```python
from build123d import *

# Parameters (mm, degrees)
SKETCH1_R           = 4.15
BOSS_EXTRUDE1_DEPTH = 27
BOSS_EXTRUDE2_DEPTH = 49
SKETCH3_W           = 7.137224295
SKETCH3_H           = 7.139279227
BOSS_EXTRUDE3_DEPTH = 49
SKETCH4_R           = 2
CUT_EXTRUDE1_DEPTH  = 51
FILLET1_R           = 3
SKETCH5_W           = 7.156865167
SKETCH5_H           = 37
CUT_EXTRUDE2_DEPTH  = 7.139279
SKETCH7_W           = 36.574972609
SKETCH7_H           = 48.532858444
CUT_EXTRUDE3_DEPTH  = 51
SKETCH8_W           = 4
SKETCH8_H           = 11
BOSS_EXTRUDE4_DEPTH = 49
SKETCH10_R          = 3.175
CUT_EXTRUDE4_DEPTH  = 49


with BuildPart() as part:
    # Sketch1 → Boss-Extrude1 (new body)
    with BuildSketch(Plane(origin=(0, 0, 0), x_dir=(1, 0, 0), z_dir=(0, 1, 0))):
        with BuildLine():
            Line((-6.5, 48.7), (-6.5, 0))
            ThreePointArc((-6.5, 0), (0, -6.5), (6.5, 0))
            Line((6.5, 0), (6.5, 48.7))
            ThreePointArc((6.5, 48.7), (0, 55.2), (-6.5, 48.7))
        make_face()
        with Locations(Location((0, 0, 0), (0, 0, 270))):  # turned: the seam where the file's is
            Circle(SKETCH1_R, mode=Mode.SUBTRACT)
        with Locations(Location((0, 48.7, 0), (0, 0, 270))):  # turned: the seam where the file's is
            Circle(SKETCH1_R, mode=Mode.SUBTRACT)
    extrude(amount=BOSS_EXTRUDE1_DEPTH)

    # Sketch2 → Boss-Extrude2 (add)
    with BuildSketch(Plane.XY):
        with BuildLine():
            Line((6.5, 27), (6.5, 0))
            Line((6.5, 0), (15.568570347, -6.685733343))
            ThreePointArc((15.568570347, -6.685733343), (43.70403904, -11.497551626), (60.435084664, 11.628846841))
            Line((60.435084664, 11.628846841), (62.638339389, 10.782838022))
            Line((62.638339389, 10.782838022), (62.638339389, 13.5))
            Line((62.638339389, 13.5), (57.5, 13.5))
            ThreePointArc((57.5, 13.5), (26.437253933, -9.437253933), (13.656865167, 27))
            Line((13.656865167, 27), (6.5, 27))
        make_face()
    extrude(amount=-BOSS_EXTRUDE2_DEPTH)

    # Sketch3 → Boss-Extrude3 (add)
    with BuildSketch(Plane.XY):
        with Locations((10.068612148, 30.569639614)):
            Rectangle(SKETCH3_W, SKETCH3_H)
    extrude(amount=-BOSS_EXTRUDE3_DEPTH)

    # Sketch4 → Cut-Extrude1 (cut)
    with BuildSketch(Plane.XY):
        with Locations((10.068612147, 30.569639613)):
            Circle(SKETCH4_R)
    extrude(amount=-CUT_EXTRUDE1_DEPTH, mode=Mode.SUBTRACT)

    # Fillet1
    fillet1_edges = [part.edges().sort_by_distance(p)[0] for p in [
        (6.5, 34.139279227, -24.5),
        (13.637224295, 34.139279227, -24.5),
    ]]
    fillet(fillet1_edges, radius=FILLET1_R)

    # Sketch5 → Cut-Extrude2 (cut)
    with BuildSketch(Plane(origin=(0, 34.139279227, 0), x_dir=(1, 0, 0), z_dir=(0, 1, 0))):
        with Locations((10.078432583, 24.5)):
            Rectangle(SKETCH5_W, SKETCH5_H)
    extrude(amount=-CUT_EXTRUDE2_DEPTH, mode=Mode.SUBTRACT)

    # Sketch7 → Cut-Extrude3 (cut)
    with BuildSketch(Plane.XY):
        with Locations((51.787486304, 3.889520552)):
            Rectangle(SKETCH7_W, SKETCH7_H)
    extrude(amount=-CUT_EXTRUDE3_DEPTH, mode=Mode.SUBTRACT)

    # Sketch8 → Boss-Extrude4 (add)
    with BuildSketch(Plane.XY):
        with Locations((31.5, -16)):
            Rectangle(SKETCH8_W, SKETCH8_H)
    extrude(amount=-BOSS_EXTRUDE4_DEPTH)

    # Sketch10 → Cut-Extrude4 (cut)
    with BuildSketch(Plane.ZY.offset(-29.5)):
        with Locations(Location((-36.75, -17.351029923, 0), (0, 0, 270))):  # turned: the seam where the file's is
            Circle(SKETCH10_R)
        with Locations(Location((-12.25, -17.351029923, 0), (0, 0, 270))):  # turned: the seam where the file's is
            Circle(SKETCH10_R)
    extrude(amount=-CUT_EXTRUDE4_DEPTH, mode=Mode.SUBTRACT)


solid = part.part
```
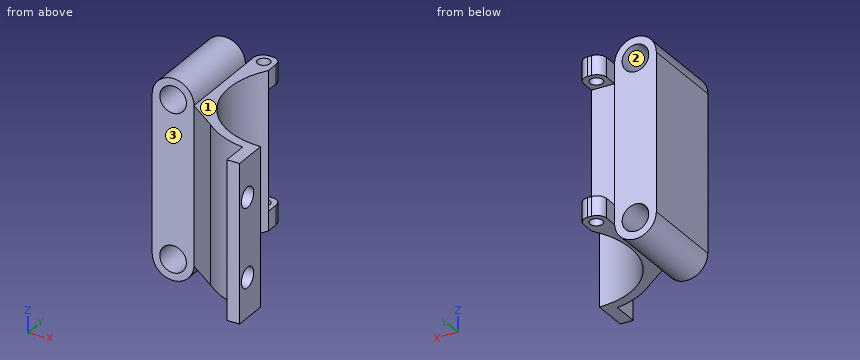
CAD build for the part. Positions are in the model's coordinates, mm. Face numbers are marked on the shaded views. Round coordinates to 2 decimals unless told otherwise and drop trailing zeros. Order: outer loops, then holes, each group sorted by start corner. A loop starts at its lowest first (then second) coordinate and runs counter-clockwise, first axis right, second up.
Q1. Slice it at C-C (y = 8). Write the cut outline in (x, z), and give its area (3 significant figures).
Q2. Slice it at D-D (x = 30.5). Write the cut outline in (y, z) (3 decimals).
Q3. Wall check: L1, parallel to Z at x = 0.5, y = 10.5; L2, parallel to Z at x = 2, y = 24; L3, parallel to X at y = 6, z = -49.5. Give the ranges that are in metal, low to high.
Q4. Drop flat-ended pins along their axis: pin 1 (11 mm diameter, centred on x = 0, z = 0, fed in from +Y); pin 2 (10 mm diameter, centred on x = 6.5, y = -4.5, fed in from +Z); pin 3 (10.5 mm diameter, centred on x = 3, z = -13, fed in from -Y). Give the stop position or say it passes through.
Q5. Slice it at B-B (x = -1). Write the cut outline in (y, z), and give its area (3 significant figures).
Q6. Slice it at A-A (z = -36.75). Write the cut outline in (x, y), and give its area (3 significant figures).
Q7. Two-plate mould, pull along Z, no slides. Class the marked faces 1, 2 and 3: pulls with the +Z half, pulls with the -Z half, needs draft (parallel to the pull), parting line crosses it, or undercut.
Results below:
1. outline: (-6.5, -48.7) arc R6.5 ccw to (6.5, -48.7) - (6.5, -49) - (10.14, -49) - (10.14, 0) - (6.5, 0) arc R6.5 ccw to (-6.5, 0) - close; hole circle Ø8.3 at (0, -48.7); hole circle Ø8.3 at (0, 0)
1. area: 836 mm2
2. outline: (-21.5, -49) - (-10.312, -49) - (-10.312, 0) - (-21.5, 0) - close; hole circle Ø6.35 at (-17.351, -36.75); hole circle Ø6.35 at (-17.351, -12.25)
3. L1: z = -55.18 to -52.82, -44.58 to -4.12, 4.12 to 6.48
3. L2: z = -54.88 to -52.34, -45.06 to -3.64, 3.64 to 6.18
3. L3: x = -6.45 to -4.07, 4.07 to 6.45
4. pin 1: stops at y = 27
4. pin 2: stops at z = 4.86
4. pin 3: stops at y = -1.29
5. outline: (0, -55.12) - (27, -55.12) - (27, -52.73) - (0, -52.73) - close; (0, -44.67) - (27, -44.67) - (27, -4.03) - (0, -4.03) - close; (0, 4.03) - (27, 4.03) - (27, 6.42) - (0, 6.42) - close
5. area: 1,230 mm2
6. outline: (-6.5, 0) - (6.5, 0) - (15.57, -6.69) arc R27 ccw to (29.5, -13.2) - (29.5, -14.18) - (33.5, -14.18) - (33.5, -10.5) arc R24 cw to (13.66, 27) - (-6.5, 27) - close; (29.5, -21.5) - (33.5, -21.5) - (33.5, -20.53) - (29.5, -20.53) - close
6. area: 563 mm2
7. face 1: pulls with the +Z half
7. face 2: undercut
7. face 3: needs draft
